Here's the drawing with two shaded views (mm, measured from the low corner). I have some questions. A direction names the side the tool comes from. Round coordinates to 2 decimals unless told otherwise and drop trailing zeros. Write each loop counter-clockwise with the first axis right and the second up, starting at its lowest first coordinate (ties: lowest second). Pieces come first, ordered by that corner, then holes. Notation, with made-up numbers: M 4.25,9.5 L 43.25,9.5 A28 cw 43.25,46.5 Z; hole C -33,13 d8. An arc over 180 degrees is marked long. Write item = value, one per line. Start each with the question number.
(1) I need wall thicknesses on line 1 along Y through (x, z) = (3, 57); line 2 along Z through (x, y) = (57, 140.5); line 3 along Z through (x, y) = (3.75, 190.5). Which ranges of each line are inside material? Lowest first, please.
(2) I want a section at B-B (y = 38.1). Give the number of separate pieces and of enclosed holes in the cut face, and give its area (3 significant figures).
(3) I want a section at C-C (z = 32.5). List the corners of the cut face in (x, y) for me.
(4) I want a section at A-A (x = 57.15). List the corners of the cut face in (y, z) for me.
(5) On a 3-axis mill with a long thin cutter (end or side, diameter ignored), from which of +Z, -Z, +X, -X, +Y, -Y can I reach the whole of each face in a straight line? I mean the marked faces 1 and 2. Say none if no direction works.
(6) Will these pins go through, and if not, where does the flat tip stop? pin 1 Ø12 at (x, y) = (67, 60.5) entering from +Z; pin 2 Ø21 at (y, z) = (191, 67.5) entering from +X.
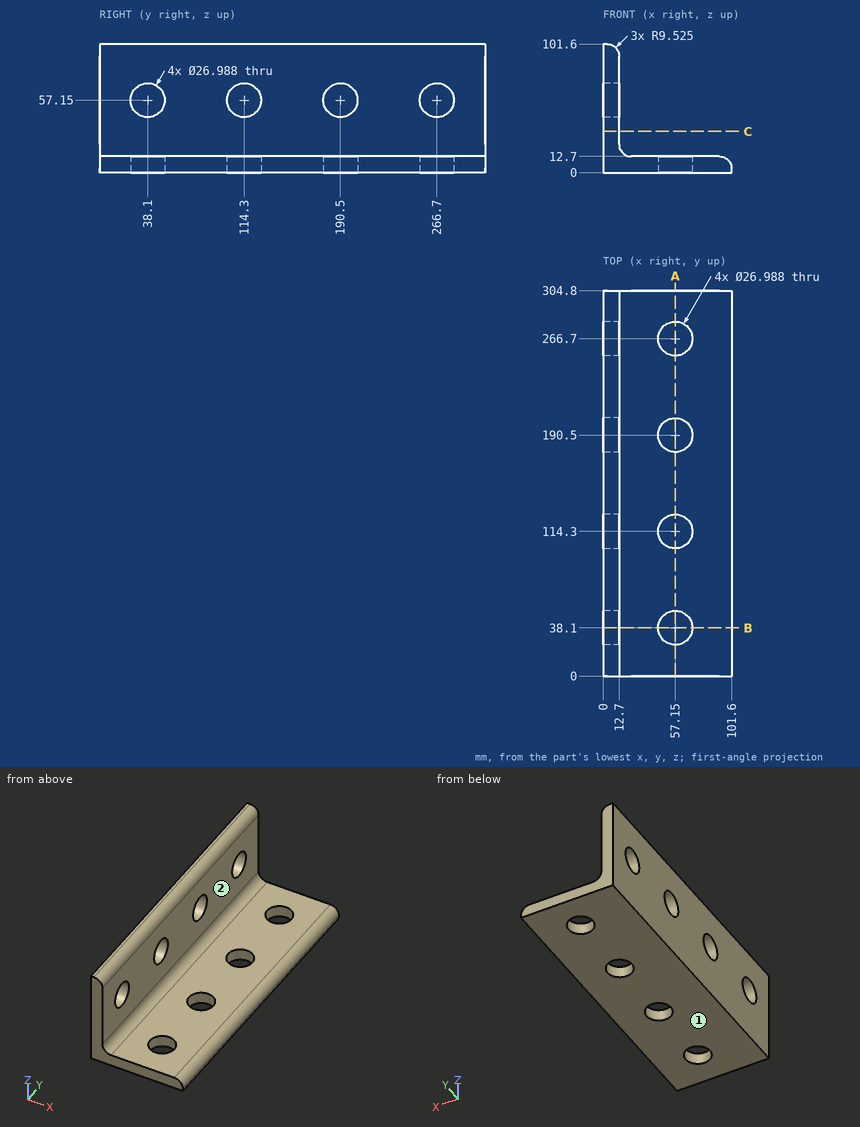
Returned:
q1.line_1 = 0 to 24.61, 51.59 to 100.81, 127.79 to 177.01, 203.99 to 253.21, 280.19 to 304.8
q1.line_2 = 0 to 12.7
q1.line_3 = 0 to 43.66, 70.64 to 101.58
q2.separate_pieces = 3
q2.enclosed_holes = 0
q2.area = 1,710 mm²
q3.outline = M 0,0 L 12.7,0 L 12.7,304.8 L 0,304.8 Z
q4.outline = M 0,0 L 24.61,0 L 24.61,12.7 L 0,12.7 Z; M 51.59,0 L 100.81,0 L 100.81,12.7 L 51.59,12.7 Z; M 127.79,0 L 177.01,0 L 177.01,12.7 L 127.79,12.7 Z; M 203.99,0 L 253.21,0 L 253.21,12.7 L 203.99,12.7 Z; M 280.19,0 L 304.8,0 L 304.8,12.7 L 280.19,12.7 Z
q5.face_1 = -Z, +X, -X, +Y, -Y
q5.face_2 = +Z, +X, +Y, -Y
q6.pin_1 = 12.7
q6.pin_2 = 12.7
